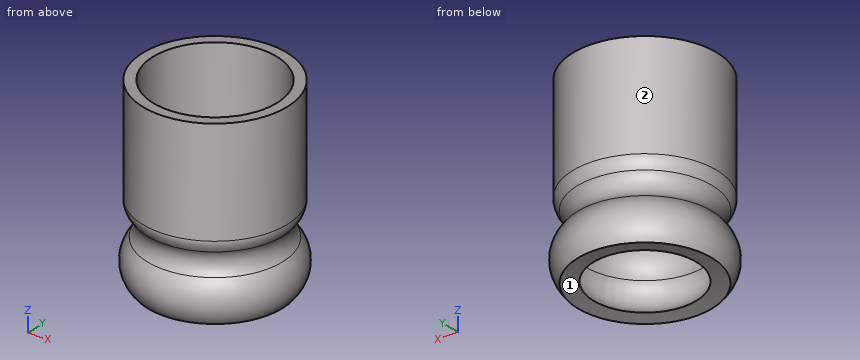
```python
from build123d import *


with BuildPart() as part:
    # 草图2 → 旋转1 (revolve)
    with BuildSketch(Plane(origin=(0, 0, 0), x_dir=(1, 0, 0), z_dir=(0, 1, 0))):
        with BuildLine():
            ThreePointArc((13.104115055, 22.770530099), (12.25, 25), (13.104115055, 27.229469901))
            ThreePointArc((13.104115055, 27.229469901), (14.639719012, 31.287170848), (13.038257502, 35.319333731))
            Line((13.038257502, 35.319333731), (10, 35))
            ThreePointArc((10, 35), (12.519423129, 32.212719337), (11.616049309, 28.565755924))
            ThreePointArc((11.616049309, 28.565755924), (10.25, 25), (11.616049309, 21.434244076))
            ThreePointArc((11.616049309, 21.434244076), (11.900727305, 20.968651416), (12, 20.432029558))
            Line((12, 20.432029558), (12, 0))
            Line((12, 0), (14, 0))
            Line((14, 0), (14, 20.432029558))
            ThreePointArc((14, 20.432029558), (13.768363711, 21.684147226), (13.104115055, 22.770530099))
        make_face()
    revolve(axis=Axis((0, 0, 0), (0, 0, -1)))


solid = part.part
```
Design review of the part built by this model. Coordinates are the model's own, in mm. Face numbers are marked on the shaded views. Round coordinates to 2 decimals unless told otherwise and drop trailing zeros. Write each loop counter-clockwise with the first axis right and the second up, starting at its lowest first coordinate (ties: lowest second). Pieces come first, ordered by that corner, then holes. Notation, with made-up numbers: (61.5, 50) -> (89.5, 50) arc R32 cw to (89.5, 88) -> close; hole circle Ø7 at (-23.5, 9.5). An arc over 180 degrees is marked (long way). Answer in a Markdown table with one row per item.
Q1. Take a section at C-C, the plane z = -17.5. State the section outline as (x, y) points.
The answers:
| item | result |
|---|---|
| outline | circle Ø28 at (0, 0); hole circle Ø24 at (0, 0) |
Q2. To check wall thickness, follow L1, parallel to X at y = 0.5, z = -16; L2, parallel to Y at x = 0, z = -14.75; L3, parallel to X at y = 4.25, z = -19. State the ranges of each line that lie inside material, in increasing order. Write a range as [from, to].
The answers:
| item | result |
|---|---|
| L1 | [-13.99, -11.99], [11.99, 13.99] |
| L2 | [-14, -12], [12, 14] |
| L3 | [-13.34, -11.22], [11.22, 13.34] |
Q3. Take a section at A-A, the plane y = 0. State the section outline as (x, z) points.
The answers:
| item | result |
|---|---|
| outline | (-14, -20.43) arc R3.5 ccw to (-13.1, -22.77) arc R3.34 cw to (-13.1, -27.23) arc R6 ccw to (-13.04, -35.32) -> (-10, -35) arc R4 cw to (-11.62, -28.57) arc R5.34 ccw to (-11.62, -21.43) arc R1.5 cw to (-12, -20.43) -> (-12, 0) -> (-14, 0) -> close; (10, -35) -> (13.04, -35.32) arc R6 ccw to (13.1, -27.23) arc R3.34 cw to (13.1, -22.77) arc R3.5 ccw to (14, -20.43) -> (14, 0) -> (12, 0) -> (12, -20.43) arc R1.5 cw to (11.62, -21.43) arc R5.34 ccw to (11.62, -28.57) arc R4 cw to start |
Q4. Draft analysis for pull direction X (two halves, no side actions). For the marked faces 1 and 2, state which applies: +X half, -X half, draft (parallel to the pull), parting line (faces both ways), or undercut.
The answers:
| item | result |
|---|---|
| face 1 | undercut |
| face 2 | parting line |
Q5. Clearance check with flat-ended pins moving along their axes: pin 1 Ø3 at (x, z) = (6.5, -9.5) entering from +Y; pin 2 Ø1 at (x, y) = (7.5, 7) entering from -Z; pin 3 Ø8 at (y, z) = (5.5, -9) entering from +X; pin 4 Ø14.5 at (x, y) = (0, 0) entering from -Z. State where each tip first meets the part, or that it passes through.
The answers:
| item | result |
|---|---|
| pin 1 | y = 13.08 |
| pin 2 | z = -35.08 |
| pin 3 | x = 13.92 |
| pin 4 | through |
Q6. Take a section at D-D, the plane z = -22. State the section outline as (x, y) points.
The answers:
| item | result |
|---|---|
| outline | circle Ø27.26 at (0, 0); hole circle Ø22.35 at (0, 0) |
